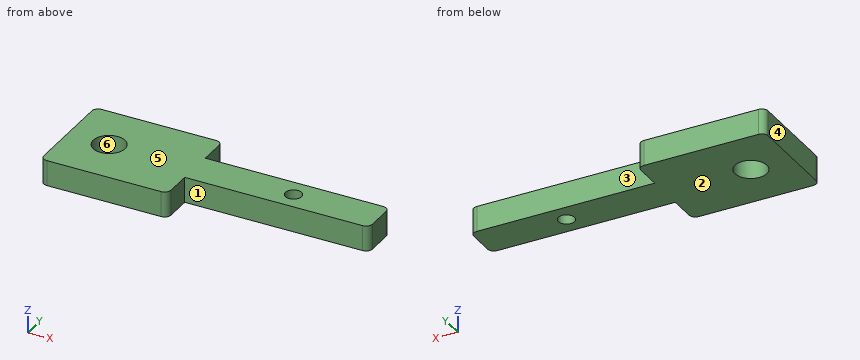
from build123d import *

# Parameters (mm, degrees)
F1_DEPTH = 6.35
F2_D     = 7.9375
F3_D     = 4.0386


with BuildPart() as f1:
    # F0 (on Top) → F1 (new body)
    with BuildSketch(Plane.XY):
        with BuildLine():
            Line((30.1625, 0), (1.5875, 0))
            ThreePointArc((1.5875, 0), (0.4649679849, -0.4649679849), (0, -1.5875))
            Line((0, -1.5875), (0, -23.8125))
            ThreePointArc((0, -23.8125), (0.4649679849, -24.9350320151), (1.5875, -25.4))
            Line((1.5875, -25.4), (30.1625, -25.4))
            ThreePointArc((30.1625, -25.4), (31.2850320151, -24.9350320151), (31.75, -23.8125))
            Line((31.75, -23.8125), (31.75, -17.4625))
            Line((31.75, -17.4625), (76.1873, -17.4625))
            ThreePointArc((76.1873, -17.4625), (77.3098320151, -16.9975320151), (77.7748, -15.875))
            Line((77.7748, -15.875), (77.7748, -9.525))
            ThreePointArc((77.7748, -9.525), (77.3098320151, -8.4024679849), (76.1873, -7.9375))
            Line((76.1873, -7.9375), (31.75, -7.9375))
            Line((31.75, -7.9375), (31.75, -1.5875))
            ThreePointArc((31.75, -1.5875), (31.2850320151, -0.4649679849), (30.1625, 0))
        make_face()
    extrude(amount=F1_DEPTH)

    # F2 (through all)
    with Locations(Plane(origin=(0, 0, 0), x_dir=(1, 0, 0), z_dir=(0, 0, -1))):
        with Locations((10.3124, 12.7)):
            Hole(F2_D / 2)

    # F3 (through all)
    with Locations(Plane(origin=(0, 0, 0), x_dir=(1, 0, 0), z_dir=(0, 0, -1))):
        with Locations((56.3626, 12.7)):
            Hole(F3_D / 2)


solid = f1.part
Input: part model. Units: mm. Frame: model coordinates. Face numbers are marked on the shaded views. A direction names the side the tool comes from. Give positions to 0.01 mm unless a question says otherwise; leave off trailing zeros. Order: outer loops, then holes, each group sorted by start corner. A loop starts at its lowest first (then second) coordinate and runs counter-clockwise, first axis right, second up. Notation, with made-up numbers: (29, 67) - (64, 67) arc R3 ccw to (64, 72) - close; hole circle Ø10 at (-12.5, -6). An arc over 180 degrees is marked (long way). Answer as a JSON object with one key per item and string values. Group by question number.
Q1. Line query: probe 1 along X at (y, z) = (-11, 3.5); probe 2 along Y at (x, z) = (47, 1.5); probe 3 along Y at (x, z) = (11.5, 2.5). Output: solid intervals per line, ascending.
Q2. Cut plane B-B, the plane x = 11.5. Output: boundary loops of the cut face in (y, z), then the cut area to 3 significant figures.
Q3. Cut plane D-D, the plane y = -20.75. Output: boundary loops of the cut face in (x, z).
Q4. Cut plane A-A, the plane y = -12.7. Output: boundary loops of the cut face in (x, z).
Q5. Mould query, pull axis X, two halves, no side actions, for the marked faces 4, 5 and 6. Classes: pulls with the +X half, pulls with the -X half, needs draft (parallel to the pull), parting line crosses it, or undercut.
Q6. Set-up query: the marked faces 1, 2 and 3. Return all of +Z, -Z, +X, -X, +Y, -Y with unobstructed straight access to the full face (end or side cutting, diameter ignored); none if empty.
Q7. Cut plane C-C, the plane z = 1. Count the separate pieces of the cut face and the enclosed holes in it, then the cut area to 3 significant figures.
Q8. First-contact query: pin 1 Ø5 at (x, y) = (10.31, -12.7) entering from +Z; pin 2 Ø1.9 at (x, z) = (57.5, 4.5) entering from +Y; pin 3 Ø1.5 at (x, z) = (50.5, 5) entering from -Y; pin 4 Ø1.9 at (y, z) = (-20, 3) entering from +X. Flat tips, straight axial feed; report the tip coordinate or a pass-through.
Results:
{
 "1": {"probe 1": "0 to 6.73, 13.9 to 55.27, 57.45 to 77.77", "probe 2": "-17.46 to -7.94", "probe 3": "-25.4 to -16.49, -8.91 to 0"},
 "2": {"outline": "(-25.4, 0) - (-16.49, 0) - (-16.49, 6.35) - (-25.4, 6.35) - close; (-8.91, 0) - (0, 0) - (0, 6.35) - (-8.91, 6.35) - close", "area": "113 mm^2"},
 "3": {"outline": "(0, 0) - (31.75, 0) - (31.75, 6.35) - (0, 6.35) - close"},
 "4": {"outline": "(0, 0) - (6.34, 0) - (6.34, 6.35) - (0, 6.35) - close; (14.28, 0) - (54.34, 0) - (54.34, 6.35) - (14.28, 6.35) - close; (58.38, 0) - (77.77, 0) - (77.77, 6.35) - (58.38, 6.35) - close"},
 "5": {"face 4": "pulls with the -X half", "face 5": "needs draft", "face 6": "undercut"},
 "6": {"face 1": "+Z, -Z, +X, -Y", "face 2": "-Z, +X, -X, +Y, -Y", "face 3": "+Z, -Z, +X, +Y"},
 "7": {"separate pieces": "1", "enclosed holes": "2", "area": "1,180 mm^2"},
 "8": {"pin 1": "through", "pin 2": "y = -7.94", "pin 3": "y = -17.46", "pin 4": "x = 31.75"}
}
